Autodesk Inventor part; units mm, degrees
ref_plane "YZ Plane" through (0, 0, 0) normal (1, 0, 0) x (0, 1, 0)
ref_plane "XZ Plane" through (0, 0, 0) normal (0, 1, 0) x (-1, 0, 0)
ref_plane "XY Plane" through (0, 0, 0) normal (0, 0, 1) x (1, 0, 0)
sketch "Эскиз1" plane through (0, 0, 0) normal (0, 0, 1) x (1, 0, 0)
  line L0 (2, 0) -> (12, 0)
  line L1 (14, 2) -> (14, 14)
  line L2 (14, 14) -> (0, 14)
  line L3 (0, 14) -> (0, 2)
  circle A0 centre (7, 7) radius 1.5
  arc A1 (0, 2) -> (2, 0) centre (2, 2) ccw
  arc A2 (12, 0) -> (14, 2) centre (12, 2) ccw
  point P0 (0, 0)
  point P1 (14, 0)
  dimension "d0" = 14
  dimension "d1" = 14
  dimension "d2" = 3
  dimension "d5" = 2
extrude "Выдавливание1" add sketch "Эскиз1" along normal blind 1.5
sketch "Эскиз2" plane through (0, 0, 1.5) normal (0, 0, 1) x (1, 0, 0)
  line L0 (14, 2) -> (14, 14)
  line L1 (14, 14) -> (0, 14)
  line L2 (0, 14) -> (0, 12.5)
  line L3 (0, 12.5) -> (14, 12.5)
  line L4 (14, 12.5) -> (14, 14)
  point P0 (0, 0)
  dimension "d6" = 14
  dimension "d7" = 1.5
extrude "Выдавливание2" add sketch "Эскиз2" along normal blind 12.5
fillet "Сопряжение1" radius 2 4 edges at (0, 13.25, 14) (14, 13.25, 14) (7, 12.5, 1.5) (7, 14, 0)
sketch "Эскиз3" plane through (0, 12.5, 3.5) normal (0, -1, 0) x (1, 0, 0)
  line L0 (2, 10.5) -> (12, 10.5)
  line L1 (7, 10.5) -> (7, 9.5925)
  line L2 (0, 0) -> (0, 8.5)
  line L3 (0, 4.25) -> (2.1841, 4.25)
  circle A0 centre (7, 4.25) radius 1.5
  point P0 (0, -3.5)
  dimension "d11" = 3
extrude "Выдавливание3" cut sketch "Эскиз3" against normal blind 12.5
properties part number "угол 25-26"
Build history of the part. All positions in model axes, mm. A direction names the side the tool comes from. Coordinates: 2 decimals unless noted, no trailing zeros. Order: outer loops, then holes, each group sorted by start corner. A loop starts at its lowest first (then second) coordinate and runs counter-clockwise, first axis right, second up. Notation, with made-up numbers: M -35.5,85.25 L -28.5,85.25 A27 cw -28.5,114.25 Z; hole C -2.5,-22 d7. An arc over 180 degrees is marked long. One line per question, with ' | ' between items. Start each with the question number.
Q1. Saw through at D-D (x = 3.5). List the corners of the cut face in (y, z), then the cut area to 4 significant figures.
Q2. Saw through at C-C (y = 7). List the corners of the cut face in (x, z).
Q3. 3-axis set-ups, long thin cutter, end or side, ignore diameter. For faces 5 (the face through (7, 12.5, 10)), 6 (the face through (7, 0, 1)): which of +Z, -Z, +X, -X, +Y, -Y reach the whole face in a straight line?
Q4. Probe L1, parallel to Y at x = 13, z = 13.5; L2, parallel to Z at x = 7, y = 13; L3, parallel to Z at x = 7.75, y = 3. List the from-to ranges inside material, lowest first. Write a range as from..to.
Q5. Flat gauge pins, fed straight in: pin 1 Ø5 at (x, z) = (7, 8) entering from -Y; pin 2 Ø3.5 at (x, y) = (7, 7) entering from -Z. Where does each tip first touch, or does it go through?
Q6. Saw through at A-A (x = 7). List the corners of the cut face in (y, z).
Q7. Two-plate mould, pull along X, no slides. Class faces 1 (the face through (14, 11.5, 1.5)), 2 (the face through (0.6, 13.24, 13.43)), 3 (the face through (5.8, 7.9, 0.7)), 4 (the face through (5.81, 13.24, 6.84)): +X half, -X half, draft (parallel to the pull), parting line (faces both ways), or undercut.
Q8. Saw through at B-B (z = 7.75). List the corners of the cut face in (x, y).
Check values:
1) outline: M 0,0 L 12,0 A2 ccw 14,2 L 14,14 L 12.5,14 L 12.5,3.5 A2 cw 10.5,1.5 L 0,1.5 Z | area: 39.75 mm2
2) outline: M 0,0 L 5.5,0 L 5.5,1.5 L 0,1.5 Z; M 8.5,0 L 14,0 L 14,1.5 L 8.5,1.5 Z
3) face 5: +Z, +X, -X, -Y | face 6: +Z, -Z, +X, -X, -Y
4) L1: y = 12.5..14 | L2: z = 0.27..6.25, 9.25..14 | L3: z = 0..1.5
5) pin 1: stops at y = 12.5 | pin 2: stops at z = 0
6) outline: M 0,0 L 5.5,0 L 5.5,1.5 L 0,1.5 Z; M 8.5,0 L 12,0 A2 ccw 14,2 L 14,6.25 L 12.5,6.25 L 12.5,3.5 A2 cw 10.5,1.5 L 8.5,1.5 Z; M 12.5,9.25 L 14,9.25 L 14,14 L 12.5,14 Z
7) face 1: +X half | face 2: -X half | face 3: undercut | face 4: undercut
8) outline: M 0,12.5 L 5.5,12.5 L 5.5,14 L 0,14 Z; M 8.5,12.5 L 14,12.5 L 14,14 L 8.5,14 Z
